Autodesk Inventor part; units mm, degrees
ref_plane "YZ Plane" through (0, 0, 0) normal (1, 0, 0) x (0, 1, 0)
ref_plane "XZ Plane" through (0, 0, 0) normal (0, 1, 0) x (-1, 0, 0)
ref_plane "XY Plane" through (0, 0, 0) normal (0, 0, 1) x (1, 0, 0)
ref_plane "Work Plane3" through (0, 0, 4) normal (0, 0, 1) x (1, 0, 0)
ref_plane "Work Plane4" through (0, 0, 11) normal (0, 0, -1) x (-1, 0, 0)
sketch "Sketch7" plane through (0, 0, 4) normal (0, 0, 1) x (1, 0, 0)
  circle A0 centre (0, 0) radius 3.5
  circle A1 centre (0, 0) radius 7.955
  dimension "d17" = 7
  dimension "d18" = 15.91
extrude "Extrusion5" add sketch "Sketch7" along normal blind 2.7 contours A0 | A1
sketch "Sketch8" plane through (0, 0, 6.7) normal (0, 0, 1) x (1, 0, 0)
  circle A0 centre (0, 0) radius 6.25
  dimension "d21" = 12.5
extrude "Extrusion6" add sketch "Sketch8" along normal up to surface (4.3 mm away)
sketch "Sketch9" plane through (0, 0, 11) normal (0, 0, 1) x (1, 0, 0)
  circle A0 centre (0, 0) radius 10.3925
  dimension "d24" = 20.785
extrude "Extrusion7" add sketch "Sketch9" along normal blind 11
sketch "Sketch10" plane through (0, 0, 22) normal (0, 0, 1) x (1, 0, 0)
  circle A0 centre (0, 0) radius 10.3925
  line L0 (-4.1858, 7.25) -> (4.1858, 7.25)
  line L1 (4.1858, 7.25) -> (8.3716, 0)
  line L2 (8.3716, 0) -> (4.1858, -7.25)
  line L3 (4.1858, -7.25) -> (-4.1858, -7.25)
  line L4 (-4.1858, -7.25) -> (-8.3716, 0)
  line L5 (-8.3716, 0) -> (-4.1858, 7.25)
  line L6 (0, 0) -> (4.1858, 7.25) construction
  line L7 (0, 0) -> (8.3716, 0) construction
  line L8 (0, 0) -> (-4.1858, -7.25) construction
  line L9 (-14.5495, 0) -> (14.5495, 0)
  dimension "d27" = 14.5
extrude "Extrusion8" cut sketch "Sketch10" against normal blind 9.4 contours L9 L5 L0 L1 | L2 L3 L4 L9
properties part number "BlankSmallGearOutput"
Source: CAD feature listing. Evaluate the final solid. Frame: model axes, mm. A direction names the side the tool comes from. Coordinates: 2 decimals unless noted, no trailing zeros. Write each loop counter-clockwise with the first axis right and the second up, starting at its lowest first coordinate (ties: lowest second). Pieces come first, ordered by that corner, then holes. Notation, with made-up numbers: (33.5, 62) - (66.5, 62) arc R25 cw to (66.5, 100) - close; hole circle Ø3 at (88, 89.5). An arc over 180 degrees is marked (long way). Answer as a JSON object with one key per item and string values.
Q1. Material intervals for line 1 (Z direction, x = 6.75, y = -2.5); line 2 (Z direction, x = 0, y = -7.5); line 3 (Z direction, x = 4.5, y = 0.25), sorted ascending. Write a range as [from, to].
Ans:
{"line 1": "z = [4, 6.7], [11, 12.6]", "line 2": "z = [4, 6.7], [11, 22]", "line 3": "z = [4, 12.6]"}
Q2. Section query D-D, the plane x = -2.75. Output: boundary loops of the cut face in (y, z).
Ans:
{"outline": "(-10.02, 11) - (-5.61, 11) - (-5.61, 6.7) - (-7.46, 6.7) - (-7.46, 4) - (7.46, 4) - (7.46, 6.7) - (5.61, 6.7) - (5.61, 11) - (10.02, 11) - (10.02, 22) - (7.25, 22) - (7.25, 12.6) - (-7.25, 12.6) - (-7.25, 22) - (-10.02, 22) - close"}
Q3. First-contact query: pin 1 Ø4 at (y, z) = (5.5, 19.5) entering from +X; pin 2 Ø2 at (y, z) = (5, 18) entering from +X; pin 3 Ø3 at (x, z) = (-5.5, 12.5) entering from +Y. Flat tips, straight axial feed; report the tip coordinate or a pass-through.
Ans:
{"pin 1": "stops at x = 9.79", "pin 2": "stops at x = 9.59", "pin 3": "stops at y = 9.59"}
Q4. Set-up query: faces 4 (the flat face through (-5, -4, 6.7)), 5 (the cylindrical face through (-1.724, 7.766, 5.331)), 6 (the flat face through (0, 7.25, 17)). Return all of +Z, -Z, +X, -X, +Y, -Y with unobstructed straight access to the full face (end or side cutting, diameter ignored); none if empty.
Ans:
{"face 4": "none", "face 5": "-Z", "face 6": "+Z"}
Q5. Draft query along Y for faces 1 (the flat face through (7, 0, 11)), 2 (the flat face through (6.31, -3.57, 17.37)), 3 (the cylindrical face through (-8.25, 6.32, 16.42)). Return one class per face: released by +Y, released by -Y, zero draft, split by the parting line, or undercut.
Ans:
{"face 1": "zero draft", "face 2": "undercut", "face 3": "split by the parting line"}
Q6. Section query B-B, the plane x = -6.75. Output: boundary loops of the cut face in (y, z).
Ans:
{"outline": "(-7.9, 11) - (7.9, 11) - (7.9, 22) - (2.81, 22) - (2.81, 12.6) - (-2.81, 12.6) - (-2.81, 22) - (-7.9, 22) - close; (-4.21, 4) - (4.21, 4) - (4.21, 6.7) - (-4.21, 6.7) - close"}
Q7. Section query C-C, the plane y = 2.25. Output: boundary loops of the cut face in (x, z), plus the area to 3 significant figures.
Ans:
{"outline": "(-10.15, 11) - (-5.83, 11) - (-5.83, 6.7) - (-7.63, 6.7) - (-7.63, 4) - (7.63, 4) - (7.63, 6.7) - (5.83, 6.7) - (5.83, 11) - (10.15, 11) - (10.15, 22) - (7.07, 22) - (7.07, 12.6) - (-7.07, 12.6) - (-7.07, 22) - (-10.15, 22) - close", "area": "182 mm2"}
